```python
from build123d import *

# Parameters (mm, degrees)
BOSS_EXTRUDE1_DEPTH = 10
SKETCH2_R           = 2.5
BOSS_EXTRUDE2_DEPTH = 30


with BuildPart() as part:
    # Sketch1 → Boss-Extrude1 (new body)
    with BuildSketch(Plane(origin=(0, 0, 0), x_dir=(1, 0, 0), z_dir=(0, 1, 0))):
        with BuildLine():
            Line((-0.5, -2.449489743), (-0.5, -3.449489743))
            Line((-0.5, -3.449489743), (0.5, -3.449489743))
            Line((0.5, -3.449489743), (0.5, -2.449489743))
            ThreePointArc((0.5, -2.449489743), (0, 2.5), (-0.5, -2.449489743))
        make_face()
    extrude(amount=BOSS_EXTRUDE1_DEPTH)

    # Sketch2 → Boss-Extrude2 (add)
    with BuildSketch(Plane(origin=(0, 10, 0), x_dir=(1, 0, 0), z_dir=(0, 1, 0))):
        with Locations(Location((0, 0, 0), (0, 0, 258.463040967))):
            Circle(SKETCH2_R)
    extrude(amount=BOSS_EXTRUDE2_DEPTH)


solid = part.part
```
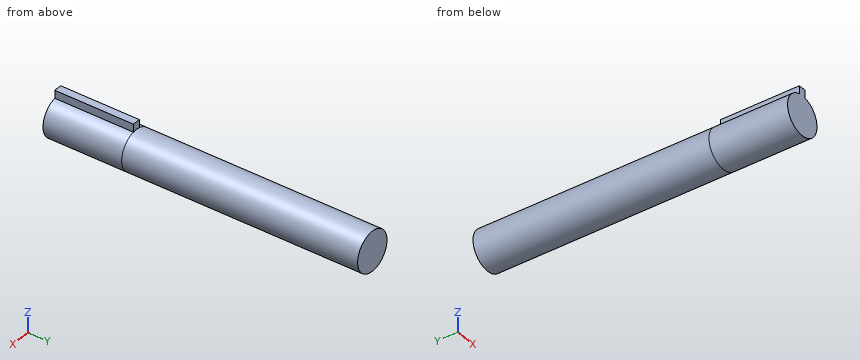
Part model, mm, in its own coordinate system. Give positions to 0.01 mm unless a question says otherwise; leave off trailing zeros. Write each loop counter-clockwise with the first axis right and the second up, starting at its lowest first coordinate (ties: lowest second). Pieces come first, ordered by that corner, then holes. Notation, with made-up numbers: (5.5, -3) -> (39.5, -3) arc R15 ccw to (39.5, 19) -> close; hole circle Ø2 at (84, 1.25). An arc over 180 degrees is marked (long way). Put each result on its own line as item: value. Start each with the question number.
Item 1: Pin check, flat tips, straight feed: pin 1 Ø0.8 at (x, z) = (0, 3) entering from +Y; pin 2 Ø3 at (x, z) = (0, -1.5) entering from -Y; pin 3 Ø2 at (y, z) = (22.5, 2.5) entering from +X. Stop position of each tip, or through.
Item 2: Cut at B-B (z = 0.8). List the corners of the cut face in (x, y).
Item 3: Cut at D-D (y = 3.5). List the corners of the cut face in (x, z), then the cut area to 3 significant figures.
Item 4: Cut at A-A (x = 0). List the corners of the cut face in (y, z).
Item 5: Wall check: L1, parallel to Y at x = 0.05, z = 3; L2, parallel to X at y = 9, z = 2.5; L3, parallel to X at y = 29.5, z = 0.2. Give the ranges that are in metal, low to high. Write a range as [from, to].
Item 6: Cut at C-C (y = 17). List the corners of the cut face in (x, z), then the cut area to 3 significant figures.
Answer list:
1. pin 1: stops at y = 10
1. pin 2: stops at y = 0
1. pin 3: stops at x = 2
2. outline: (-2.37, 0) -> (2.37, 0) -> (2.37, 40) -> (-2.37, 40) -> close
3. outline: (-0.5, 2.45) arc R2.5 ccw (long way) to (0.5, 2.45) -> (0.5, 3.45) -> (-0.5, 3.45) -> close
3. area: 20.6 mm2
4. outline: (0, -2.5) -> (40, -2.5) -> (40, 2.5) -> (10, 2.5) -> (10, 3.45) -> (0, 3.45) -> close
5. L1: y = [0, 10]
5. L2: x = [-0.5, 0.5]
5. L3: x = [-2.49, 2.49]
6. outline: circle Ø5 at (0, 0)
6. area: 19.6 mm2
